```python
from build123d import *

# Parameters (mm, degrees)
STOCK_PART1_1_DEPTH     = 2.54
CUT_EXTRUDE1_DEPTH      = 36.698530161
CUT_EXTRUDE1_DEPTH_BACK = 36.698530161
SKETCH1_R               = 3.2004


# Read off the part's stored shape, not the designer's step: Stock-Part1-1
with BuildPart() as part:
    # Stock-Part1-1 outline → Stock-Part1-1 (new body)
    with BuildSketch(Plane(origin=(0, 0, 0), x_dir=(1, 0, 0), z_dir=(0, 1, 0))):
        with BuildLine():
            ThreePointArc((-10.807074113, 22.986238255), (-11.381462581, 22.707318413), (-11.948658366, 22.414048346))
            ThreePointArc((-11.948658366, 22.414048346), (-14.055886871, 10.212199581), (-25.009365231, 4.437527549))
            ThreePointArc((-25.009365231, 4.437527549), (-25.113008503, 3.807466867), (-25.200781238, 3.175))
            Line((-25.200781238, 3.175), (-12.941946417, 3.175))
            ThreePointArc((-12.941946417, 3.175), (-9.766946417, 0), (-12.941946417, -3.175))
            Line((-12.941946417, -3.175), (-25.200781238, -3.175))
            ThreePointArc((-25.200781238, -3.175), (-25.113008503, -3.807466867), (-25.009365231, -4.437527549))
            ThreePointArc((-25.009365231, -4.437527549), (-14.055886871, -10.212199581), (-11.948658366, -22.414048346))
            ThreePointArc((-11.948658366, -22.414048346), (-11.381462581, -22.707318413), (-10.807074113, -22.986238255))
            Line((-10.807074113, -22.986238255), (-7.018885822, -11.327393516))
            ThreePointArc((-7.018885822, -11.327393516), (-3.018152425, -9.288918034), (-0.979676944, -13.289651431))
            Line((-0.979676944, -13.289651431), (-4.767865235, -24.948496169))
            ThreePointArc((-4.767865235, -24.948496169), (-4.139230233, -25.060462348), (-3.507979383, -25.156591197))
            ThreePointArc((-3.507979383, -25.156591197), (5.368871043, -16.523686022), (17.624688241, -18.290171252))
            ThreePointArc((17.624688241, -18.290171252), (18.078877786, -17.841361439), (18.521642117, -17.381276515))
            Line((18.521642117, -17.381276515), (8.604036416, -10.175714197))
            ThreePointArc((8.604036416, -10.175714197), (7.901625635, -5.740867064), (12.336472768, -5.038456283))
            Line((12.336472768, -5.038456283), (22.254078469, -12.244018601))
            ThreePointArc((22.254078469, -12.244018601), (22.554823532, -11.680750638), (22.84131474, -11.110100852))
            ThreePointArc((22.84131474, -11.110100852), (17.374031657, 0), (22.84131474, 11.110100852))
            ThreePointArc((22.84131474, 11.110100852), (22.554823532, 11.680750638), (22.254078469, 12.244018601))
            Line((22.254078469, 12.244018601), (12.336472768, 5.038456283))
            ThreePointArc((12.336472768, 5.038456283), (7.901625635, 5.740867064), (8.604036416, 10.175714197))
            Line((8.604036416, 10.175714197), (18.521642117, 17.381276515))
            ThreePointArc((18.521642117, 17.381276515), (18.078877786, 17.841361439), (17.624688241, 18.290171252))
            ThreePointArc((17.624688241, 18.290171252), (5.368871043, 16.523686022), (-3.507979383, 25.156591197))
            ThreePointArc((-3.507979383, 25.156591197), (-4.139230233, 25.060462348), (-4.767865235, 24.948496169))
            Line((-4.767865235, 24.948496169), (-0.979676944, 13.289651431))
            ThreePointArc((-0.979676944, 13.289651431), (-3.018152425, 9.288918034), (-7.018885822, 11.327393516))
            Line((-7.018885822, 11.327393516), (-10.807074113, 22.986238255))
        make_face()
    extrude(amount=STOCK_PART1_1_DEPTH)

    # Sketch1 → Cut-Extrude1 (cut, two sides: drawn at the far end of the back side and taken through both)
    with BuildSketch(Plane(origin=(0, 2.54, 0), x_dir=(1, 0, 0), z_dir=(0, 1, 0)).offset(-CUT_EXTRUDE1_DEPTH_BACK)):
        with Locations(Location((0, 0, 0), (0, 0, 270))):
            Circle(SKETCH1_R)
    extrude(amount=CUT_EXTRUDE1_DEPTH + CUT_EXTRUDE1_DEPTH_BACK, mode=Mode.SUBTRACT)


solid = part.part
```
The listing builds one solid part. Answer for the finished solid, in the listing's coordinates (mm). A direction names the side the tool comes from. Coordinates: 2 decimals unless noted, no trailing zeros. Write each loop counter-clockwise with the first axis right and the second up, starting at its lowest first coordinate (ties: lowest second). Pieces come first, ordered by that corner, then holes. Notation, with made-up numbers: (66.5, -24.75) -> (76.5, -24.75) arc R30 cw to (76.5, 14.25) -> close; hole circle Ø1 at (-24, 44.5). An arc over 180 degrees is marked (long way). Write each question's results on one line, items separated by ' | '. Start each with the question number.
1) Straight lines are drawn through the part: probe 1 along X at (y, z) = (1.3, 0); probe 2 along X at (y, z) = (2, -9.5); probe 3 along X at (y, z) = (0.4, -20.5). For each, find the intervals that lie inside material, in ascending order.
2) A cutting plane is placed at D-D (x = 6.5). Determine the outline of the cut face in (y, z), then the cut area to 3 significant figures.
3) A cutting plane is placed at A-A (z = 0). Determine the outline of the cut face in (x, y).
4) A cutting plane is placed at B-B (x = -17). Determine the outline of the cut face in (y, z) (3 decimals), then the cut area to 3 significant figures.
5) A tool of negligible diameter and unlimited length cuts with its end or side. For faces 5 (the flat face through (17.226, 1.252, 8.591)), 6 (the flat face through (-8.94, 1.25, 17.24)), 7 (the cylindrical face through (-11.4, 1.3, -22.7)), from which of +Z, -Z, +X, -X, +Y, -Y can it reach the whole face along a straight path? Write none if from no direction.
6) For a pull along Z with two mould halves and no side action, classify faces 1 (the cylindrical face through (7.86, 1.25, 5.8)), 2 (the cylindrical face through (-3.08, 1.25, 9.27)), 3 (the cylindrical face through (-25.114, 1.252, 3.799)), 4 (the flat face through (-8.89, 1.25, -17.08)) as +Z half, -Z half, draft (parallel to the pull), parting line (faces both ways), or undercut.
7) Flat-ended cylindrical pins translate along their axes: pin 1 Ø1.5 at (y, z) = (1.5, 17.5) entering from -X; pin 2 Ø10 at (x, z) = (0, 0) entering from +Y. Find the tip coordinate at first contact, or state that the pin passes through.
Values follow:
1) probe 1: -9.77 to -3.2, 3.2 to 17.37 | probe 2: -14.61 to -5.48, -2.52 to 7.92, 18.48 to 21.08 | probe 3: -11.53 to -10, -3.32 to -0.74
2) outline: (0, -16.21) -> (2.54, -16.21) -> (2.54, 16.21) -> (0, 16.21) -> close | area: 82.3 mm²
3) outline: (-9.77, 0) -> (-3.2, 0) -> (-3.2, 2.54) -> (-9.77, 2.54) -> close; (3.2, 0) -> (17.37, 0) -> (17.37, 2.54) -> (3.2, 2.54) -> close
4) outline: (0, -7.227) -> (2.54, -7.227) -> (2.54, -3.175) -> (0, -3.175) -> close; (0, 3.175) -> (2.54, 3.175) -> (2.54, 7.227) -> (0, 7.227) -> close | area: 20.6 mm²
5) face 5: +Y, -Y | face 6: +Z, +Y, -Y | face 7: -Z, -X, +Y, -Y
6) face 1: undercut | face 2: undercut | face 3: +Z half | face 4: -Z half
7) pin 1: x = -11.48 | pin 2: y = 2.54
